Source: CAD feature listing. Evaluate the final solid. Frame: model axes, mm. Face numbers are marked on the shaded views. A direction names the side the tool comes from. Round coordinates to 2 decimals unless told otherwise and drop trailing zeros. Loops run counter-clockwise (first coordinate to the right, second up) from the corner with the lowest first, then second, coordinate; pieces in that order, holes last. Notation, with made-up numbers: (31.25, 20) - (89.25, 20) arc R20 ccw to (89.25, 53) - close; hole circle Ø4 at (-7.5, 11). An arc over 180 degrees is marked (long way). Write item = value, one per line. Start each with the question number.
Autodesk Fusion 360 part; units mm, degrees
sketch "Sketch1" plane through (0, 0, 0) normal (0, 0, 1) x (1, 0, 0)
  line L0 (-15.5, 12.25) -> (15.5, 12.25)
  line L1 (15.5, 12.25) -> (15.5, -12.25)
  line L2 (15.5, -12.25) -> (-15.5, -12.25)
  line L3 (-15.5, -12.25) -> (-15.5, 12.25)
  line L4 (-15.5, 12.25) -> (15.5, -12.25) construction
  line L5 (15.5, 12.25) -> (-15.5, -12.25) construction
  dimension "d1" = 31
  dimension "d2" = 24.5
extrude "Extrude1" add sketch "Sketch1" along normal blind 10.5
shell "Shell1" thickness 1.8 removed faces 1 at (-5.1667, 4.0833, 10.5)
sketch "Sketch2" plane through (0, 0, 10.5) normal (0, 0, 1) x (-1, 0, 0)
  line L0 (13.7, 10.45) -> (13.7, -10.45)
  line L1 (13.7, -10.45) -> (-13.7, -10.45)
  line L2 (-13.7, -10.45) -> (-13.7, 10.45)
  line L3 (-13.7, 10.45) -> (13.7, 10.45)
  line L4 (15.5, 12.25) -> (-15.5, 12.25)
  line L5 (-15.5, 12.25) -> (-15.5, -12.25)
  line L6 (-15.5, -12.25) -> (15.5, -12.25)
  line L7 (15.5, -12.25) -> (15.5, 12.25)
  circle A0 centre (14.4, -11.2) radius 0.84
  line L8 (0, 0) -> (0, -2)
  line L9 (0, 0) -> (4, 0)
  circle A1 centre (-14.4, -11.2) radius 0.84
  circle A2 centre (-14.4, 11.2) radius 0.84
  circle A3 centre (14.4, 11.2) radius 0.84
  dimension "d6" = 1.68
  dimension "d7" = 11.2
  dimension "d8" = 14.4
extrude "Extrude2" add sketch "Sketch2" along normal blind 4 contours A0 | A1 | A2 | A3
fillet "Fillet1" radius 1 1 edges at (15.5, -12.25, 5.25)
fillet "Fillet1" radius 1 1 edges at (15.5, 12.25, 5.25)
fillet "Fillet1" radius 1 1 edges at (-15.5, 12.25, 5.25)
fillet "Fillet1" radius 1 1 edges at (-15.5, -12.25, 5.25)
sketch "Sketch3" plane through (-15.5, 0, 0) normal (-1, 0, 0) x (0, -1, 0)
  line L0 (11.25, 0) -> (11.25, 10.5)
  line L1 (11.25, 10.5) -> (-11.25, 10.5)
  line L2 (-11.25, 10.5) -> (-11.25, 0)
  line L3 (-11.25, 0) -> (11.25, 0)
  line L4 (0, 0) -> (0, 3.5)
  line L5 (0, 3.5) -> (0, 5)
  line L6 (-3.4, 3.5) -> (3.4, 3.5)
  line L7 (4.4, 4.5) -> (4.4, 5.5)
  line L8 (3.4, 6.5) -> (-3.4, 6.5)
  line L9 (-4.4, 5.5) -> (-4.4, 4.5)
  line L10 (-4.4, 3.5) -> (4.4, 6.5) construction
  line L11 (4.4, 3.5) -> (-4.4, 6.5) construction
  arc A0 (-3.4, 6.5) -> (-4.4, 5.5) centre (-3.4, 5.5) ccw
  arc A1 (-4.4, 4.5) -> (-3.4, 3.5) centre (-3.4, 4.5) ccw
  arc A2 (3.4, 3.5) -> (4.4, 4.5) centre (3.4, 4.5) ccw
  arc A3 (4.4, 5.5) -> (3.4, 6.5) centre (3.4, 5.5) ccw
  point P0 (0, 5)
  dimension "d19" = 3.5
  dimension "d20" = 1.5
  dimension "d21" = 3
  dimension "d22" = 8.8
  dimension "d23" = 1
extrude "Extrude3" cut sketch "Sketch3" against normal blind 6 contours L6 L7 L8 L9 A0 A1 A2 A3
fillet "Fillet2" radius 0.75 8 edges at (-15.2071, -11.9571, 0) (-15.5, 0, 0) (-15.2071, 11.9571, 0) (0, 12.25, 0) (15.2071, 11.9571, 0) (15.5, 0, 0) (15.2071, -11.9571, 0) (0, -12.25, 0)
sketch "Sketch4" plane through (0, 0, 0) normal (0, 0, -1) x (1, 0, 0)
  arc A0 (-14.5, 11.5) -> (-14.75, 11.25) centre (-14.5, 11.25) ccw
  line L0 (-14.75, 11.25) -> (-14.75, -11.25)
  arc A1 (-14.75, -11.25) -> (-14.5, -11.5) centre (-14.5, -11.25) ccw
  line L1 (-14.5, -11.5) -> (14.5, -11.5)
  arc A2 (14.5, -11.5) -> (14.75, -11.25) centre (14.5, -11.25) ccw
  line L2 (14.75, -11.25) -> (14.75, 11.25)
  arc A3 (14.75, 11.25) -> (14.5, 11.5) centre (14.5, 11.25) ccw
  line L3 (14.5, 11.5) -> (-14.5, 11.5)
  line L4 (-14.75, 0) -> (-12.7501, 0.0149)
  line L5 (7.2499, 0.0149) -> (7.2499, 8.7649)
  line L6 (7.2499, 8.7649) -> (-12.7501, 8.7649)
  line L7 (-12.7501, 8.7649) -> (-12.7501, 0.0149)
  line L8 (7.2499, 0.0149) -> (7.2499, -8.7351)
  line L9 (7.2499, -8.7351) -> (-12.7501, -8.7351)
  line L10 (-12.7501, -8.7351) -> (-12.7501, 0.0149)
  line L11 (-12.7501, -8.7351) -> (-11.7501, -8.7351)
  line L12 (-11.7501, -8.7351) -> (-11.7501, -7.7351)
  line L13 (-11.7501, -7.7351) -> (-5.2501, -7.7351)
  line L14 (-5.2501, -7.7351) -> (-5.2501, -1.2351)
  line L15 (-5.2501, -1.2351) -> (-11.7501, -1.2351)
  line L16 (-11.7501, -1.2351) -> (-11.7501, -7.7351)
  line L17 (7.2499, 8.7649) -> (6.2499, 8.7649)
  line L18 (-5.2501, -7.7351) -> (-2.2501, -7.7351)
  line L19 (-2.2501, -7.7351) -> (12.4499, -7.7351)
  line L20 (12.4499, -7.7351) -> (12.4499, -0.7351)
  dimension "d32" = 20
  dimension "d33" = 8.75
  dimension "d34" = 1
  dimension "d35" = 1
  dimension "d38" = 6.5
  dimension "d39" = 6.5
  dimension "d42" = 1
  dimension "d54" = 3
  dimension "d55" = 14.7
  dimension "d56" = 7
sketch "Sketch6" plane through (0, 0, 0) normal (0, 0, -1) x (1, 0, 0)
  arc A0 (-14.5, 11.5) -> (-14.75, 11.25) centre (-14.5, 11.25) ccw
  line L0 (-14.75, 11.25) -> (-14.75, -11.25)
  arc A1 (-14.75, -11.25) -> (-14.5, -11.5) centre (-14.5, -11.25) ccw
  line L1 (-14.5, -11.5) -> (14.5, -11.5)
  arc A2 (14.5, -11.5) -> (14.75, -11.25) centre (14.5, -11.25) ccw
  line L2 (14.75, -11.25) -> (14.75, 11.25)
  arc A3 (14.75, 11.25) -> (14.5, 11.5) centre (14.5, 11.25) ccw
  line L3 (14.5, 11.5) -> (-14.5, 11.5)
  line L4 (-15.5, 0) -> (-13.5, 0)
  line L5 (6.5, 0) -> (6.5, 8.75)
  line L6 (6.5, 8.75) -> (-13.5, 8.75)
  line L7 (-13.5, 8.75) -> (-13.5, 0)
  line L8 (-13.5, -8.75) -> (-13.5, 0)
  line L9 (6.5, -8.75) -> (-13.5, -8.75)
  line L10 (6.5, 0) -> (6.5, -8.75)
  line L11 (-13.5, 8.75) -> (-13.5, 7.75)
  line L12 (-13.5, 7.75) -> (-12.5, 7.75)
  line L13 (-12.5, 7.75) -> (-6, 7.75)
  line L14 (-6, 7.75) -> (-6, 1.25)
  line L15 (-6, 1.25) -> (-12.5, 1.25)
  line L16 (-12.5, 1.25) -> (-12.5, 7.75)
  point P0 (-13.7, 10.45)
  dimension "d57" = 2
  dimension "d58" = 10.45
  dimension "d61" = 20
  dimension "d62" = 8.75
  dimension "d63" = 1
  dimension "d64" = 1
  dimension "d65" = 6.5
  dimension "d66" = 6.5
extrude "Extrude5" cut sketch "Sketch6" against normal blind 9 contours L13 L14 L15 L16
sketch "Sketch7" plane through (15.5, 0, 0) normal (1, 0, 0) x (0, 1, 0)
  line L0 (-11.25, 0.75) -> (11.25, 0.75)
  line L1 (11.25, 0.75) -> (11.25, 10.5)
  line L2 (11.25, 10.5) -> (-11.25, 10.5)
  line L3 (-11.25, 10.5) -> (-11.25, 0.75)
  line L4 (0, 10.5) -> (0, 7.1)
  line L5 (-8.75, 7.1) -> (-8.75, 10.5)
  line L6 (-8.75, 7.1) -> (-7.75, 7.1)
  line L7 (-7.75, 7.1) -> (-0.25, 7.1)
  line L8 (-0.25, 7.1) -> (-0.25, 0.6)
  line L9 (-0.25, 0.6) -> (-7.75, 0.6)
  line L10 (-7.75, 0.6) -> (-7.75, 7.1)
  line L11 (0.25, 7.1) -> (0.25, 0.6)
  line L12 (0.25, 0.6) -> (7.75, 0.6)
  line L13 (7.75, 0.6) -> (7.75, 7.1)
  line L14 (7.75, 7.1) -> (0.25, 7.1)
  dimension "d69" = 3.4
  dimension "d70" = 8.75
  dimension "d73" = 1
  dimension "d74" = 7.5
  dimension "d75" = 6.5
extrude "Extrude6" cut sketch "Sketch7" against normal blind 19.5 contours L0 L7 L8 L10 | L0 L8 L9 L10 | L0 L11 L13 L14 | L0 L11 L12 L13
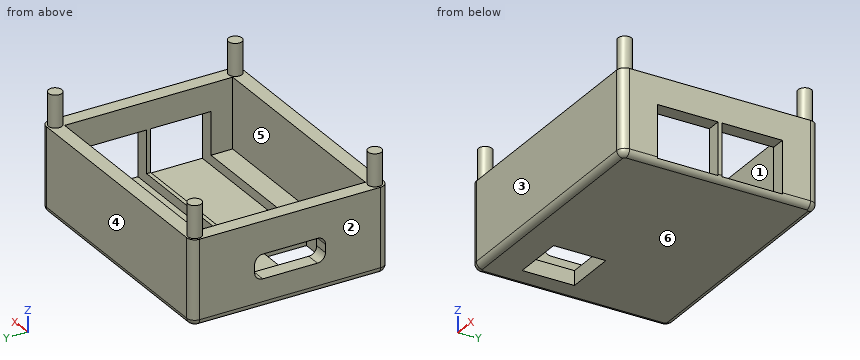
(1) Cut plane C-C (z = 7.75). Output: boundary loops of the cut face in (x, y).
(2) Access query for the marked faces 5 and 6. Directions: +Z, -Z, +X, -X, +Y, -Y. A direction counts if a zero-diameter tool reaches every point of the face in a straight line with its end or side. Return the directions, or none.
(3) Cut plane A-A (y = -6.5). Output: boundary loops of the cut face in (x, z).
(4) Cut plane B-B (y = -3). Output: boundary loops of the cut face in (x, z), and give its area (3 significant figures).
(5) Pin query (flat end, axial travel): P1, Ø5, axis at y = 3, z = 4, coming from the +X side; P2, Ø2.5, axis at y = 3, z = 5, coming from the -X side; P3, Ø4, axis at x = 2, y = 4, coming from the +Z side; P4, Ø4, axis at x = -12.5, y = 5.5, coming from the +Z side. Return the tip coordinate at first contact, or that it passes through.
(6) Mould query, pull axis Y, two halves, no side actions, for the marked faces 1, 2, 3 and 4. Classes: +Y half, -Y half, draft (parallel to the pull), parting line (faces both ways), or undercut.
(7) Cut plane D-D (z = 11). Output: boundary loops of the cut face in (x, y).
(8) Material intervals for line 1 along X through (y, z) = (9.25, 4); line 2 along Y through (x, z) = (-6.5, 3); line 3 along Z through (x, y) = (4.5, -7.5), sorted ascending. Write a range as from..to.
Solution:
q1.outline = (-15.5, -11.25) arc R1 ccw to (-14.5, -12.25) - (14.5, -12.25) arc R1 ccw to (15.5, -11.25) - (15.5, 11.25) arc R1 ccw to (14.5, 12.25) - (-14.5, 12.25) arc R1 ccw to (-15.5, 11.25) - close; hole (-13.7, -10.45) - (13.7, -10.45) - (13.7, 10.45) - (-13.7, 10.45) - close
q2.face_5 = +Z
q2.face_6 = -Z, +X, -X, +Y, -Y
q3.outline = (-15.5, 0.75) arc R0.75 ccw to (-14.75, 0) - (-12.5, 0) - (-12.5, 1.8) - (-13.7, 1.8) - (-13.7, 10.5) - (-15.5, 10.5) - close; (-6, 0) - (14.75, 0) arc R0.75 ccw to (15.48, 0.6) - (-4, 0.6) - (-4, 1.8) - (-6, 1.8) - close; (13.7, 7.1) - (15.5, 7.1) - (15.5, 10.5) - (13.7, 10.5) - close
q4.outline = (-15.5, 0.75) arc R0.75 ccw to (-14.75, 0) - (-12.5, 0) - (-12.5, 1.8) - (-13.7, 1.8) - (-13.7, 3.5) - (-15.5, 3.5) - close; (-15.5, 6.5) - (-13.7, 6.5) - (-13.7, 10.5) - (-15.5, 10.5) - close; (-6, 0) - (14.75, 0) arc R0.75 ccw to (15.48, 0.6) - (-4, 0.6) - (-4, 1.8) - (-6, 1.8) - close; (13.7, 7.1) - (15.5, 7.1) - (15.5, 10.5) - (13.7, 10.5) - close
q4.area = 36.8 mm^2
q5.P1 = -4
q5.P2 = through
q5.P3 = 0.6
q5.P4 = 10.5
q6.face_1 = undercut
q6.face_2 = draft
q6.face_3 = -Y half
q6.face_4 = +Y half
q7.outline = circle Ø1.68 at (-14.4, -11.2); circle Ø1.68 at (-14.4, 11.2); circle Ø1.68 at (14.4, -11.2); circle Ø1.68 at (14.4, 11.2)
q8.line_1 = -15.5..-13.7, 13.7..15.5
q8.line_2 = -12.25..-10.45, 10.45..12.25
q8.line_3 = 0..0.6
